Geometry check sheet. Reference: drawing and pictorial views, mm from the part's lowest x, y, z. A direction names the side the tool comes from. Give positions to 0.01 mm unless a question says otherwise; leave off trailing zeros. Write each loop counter-clockwise with the first axis right and the second up, starting at its lowest first coordinate (ties: lowest second). Pieces come first, ordered by that corner, then holes. Notation, with made-up numbers: (-24, 12) - (4, 12) arc R14 ccw to (4, 25) - close; hole circle Ø11 at (67, 73.5). An arc over 180 degrees is marked (long way). Write item = value, one per line. Start each with the question number.
(1) Thickness scan on L1, parallel to X at y = 58.5, z = 20; L2, parallel to Y at x = 11, z = 2; L3, parallel to Y at x = 54, z = 19.5. Record the ranges inside material, lowest first.
(2) Section check C-C, the plane x = 22.5. Enter the section's corners in (y, z), plus the area to 3 significant figures.
(3) Section check A-A, the plane z = 15. Enter the section's corners in (x, y), plus the area to 3 significant figures.
(4) Draft check along X on the marked faces 5, 6, 7 and 8. Enter one of: pulls with the +X half, pulls with the -X half, needs draft (parallel to the pull), parting line crosses it, or undercut.
(5) Access from +Z, -Z, +X, -X, +Y, -Y to the whole of each face (thin tool, end or side, straight path). Record for the marked faces 1, 2, 3 and 4.
(6) Section check B-B, the plane y = 48.5. Enter the section's corners in (x, z).
(7) Depth check by flat-ended pin: pin 1 Ø19.5 at (x, y) = (58.5, 24) entering from +Z; pin 2 Ø7.5 at (y, z) = (21, 9) entering from -X; pin 3 Ø6 at (x, z) = (13.5, 30) entering from +Y. Enter the tip coordinate at first touch or a pass-through.
(8) Section check D-D, the plane z = 37.5. Enter the section's corners in (x, y), plus the area to 3 significant figures.
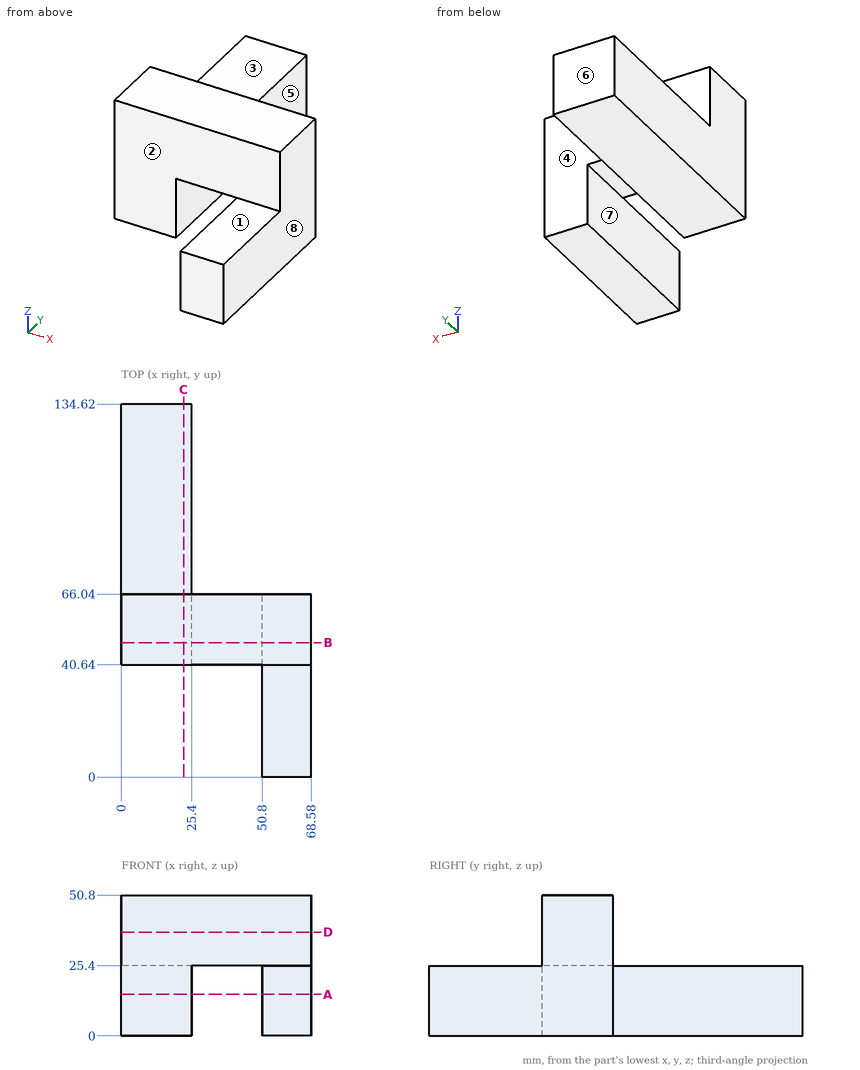
Model answer:
q1.L1 = 0 to 25.4, 50.8 to 68.58
q1.L2 = 40.64 to 134.62
q1.L3 = 0 to 66.04
q2.outline = (40.64, 0) - (134.62, 0) - (134.62, 25.4) - (66.04, 25.4) - (66.04, 50.8) - (40.64, 50.8) - close
q2.area = 3,030 mm²
q3.outline = (0, 40.64) - (25.4, 40.64) - (25.4, 134.62) - (0, 134.62) - close; (50.8, 0) - (68.58, 0) - (68.58, 66.04) - (50.8, 66.04) - close
q3.area = 3,560 mm²
q4.face_5 = undercut
q4.face_6 = needs draft
q4.face_7 = undercut
q4.face_8 = pulls with the +X half
q5.face_1 = +Z, +X, -X, -Y
q5.face_2 = +Z, -X, -Y
q5.face_3 = +Z, +X, -X, +Y
q5.face_4 = +Z, +X, +Y
q6.outline = (0, 0) - (25.4, 0) - (25.4, 25.4) - (50.8, 25.4) - (50.8, 0) - (68.58, 0) - (68.58, 50.8) - (0, 50.8) - close
q7.pin_1 = 25.4
q7.pin_2 = 50.8
q7.pin_3 = 66.04
q8.outline = (0, 40.64) - (68.58, 40.64) - (68.58, 66.04) - (0, 66.04) - close
q8.area = 1,740 mm²
